The listing builds one solid part. Answer for the finished solid, in the listing's coordinates (mm). A direction names the side the tool comes from. Give positions to 0.01 mm unless a question says otherwise; leave off trailing zeros. Loops run counter-clockwise (first coordinate to the right, second up) from the corner with the lowest first, then second, coordinate; pieces in that order, holes last. Notation, with made-up numbers: M 84,-2 L 110,-2 A19 ccw 110,14 Z; hole C 50,30 d5. An arc over 180 degrees is marked long. Return JSON: item names as keys, results as strings.
from build123d import *

# Parameters (mm, degrees)
SKETCH_2_W      = 230
SKETCH_2_H      = 60
SKETCH_2_R      = 2
EXTRUDE_1_DEPTH = 5


with BuildPart() as part:
    # 草图2 → 凸台-拉伸1 (new body)
    with BuildSketch(Plane.XY):
        Rectangle(SKETCH_2_W, SKETCH_2_H)
        with Locations((-100, 15)):
            Circle(SKETCH_2_R, mode=Mode.SUBTRACT)
        with Locations((100, 15)):
            Circle(SKETCH_2_R, mode=Mode.SUBTRACT)
        with BuildLine():
            Line((-30, 17.5), (30, 17.5))
            ThreePointArc((30, 17.5), (32.5, 15), (30, 12.5))
            Line((30, 12.5), (-30, 12.5))
            ThreePointArc((-30, 12.5), (-32.5, 15), (-30, 17.5))
        make_face(mode=Mode.SUBTRACT)
        with BuildLine():
            Line((40, -23), (100, -23))
            ThreePointArc((100, -23), (102, -25), (100, -27))
            Line((100, -27), (40, -27))
            ThreePointArc((40, -27), (38, -25), (40, -23))
        make_face(mode=Mode.SUBTRACT)
        with BuildLine():
            Line((-100, 10), (-40, 10))
            ThreePointArc((-40, 10), (-38, 8), (-40, 6))
            Line((-40, 6), (-100, 6))
            ThreePointArc((-100, 6), (-102, 8), (-100, 10))
        make_face(mode=Mode.SUBTRACT)
        with BuildLine():
            Line((-100, -10), (-40, -10))
            ThreePointArc((-40, -10), (-38, -8), (-40, -6))
            Line((-40, -6), (-100, -6))
            ThreePointArc((-100, -6), (-102, -8), (-100, -10))
        make_face(mode=Mode.SUBTRACT)
        with BuildLine():
            Line((100, -10), (40, -10))
            ThreePointArc((40, -10), (38, -8), (40, -6))
            Line((40, -6), (100, -6))
            ThreePointArc((100, -6), (102, -8), (100, -10))
        make_face(mode=Mode.SUBTRACT)
        with BuildLine():
            Line((100, 10), (40, 10))
            ThreePointArc((40, 10), (38, 8), (40, 6))
            Line((40, 6), (100, 6))
            ThreePointArc((100, 6), (102, 8), (100, 10))
        make_face(mode=Mode.SUBTRACT)
        with BuildLine():
            Line((-102.1, -17.5), (-102.1, -14.5))
            ThreePointArc((-102.1, -14.5), (-100, -12.4), (-97.9, -14.5))
            Line((-97.9, -14.5), (-97.9, -17.5))
            ThreePointArc((-97.9, -17.5), (-100, -19.6), (-102.1, -17.5))
        make_face(mode=Mode.SUBTRACT)
        with BuildLine():
            Line((102.1, -17.5), (102.1, -14.5))
            ThreePointArc((102.1, -14.5), (100, -12.4), (97.9, -14.5))
            Line((97.9, -14.5), (97.9, -17.5))
            ThreePointArc((97.9, -17.5), (100, -19.6), (102.1, -17.5))
        make_face(mode=Mode.SUBTRACT)
        with BuildLine():
            Line((-30, -17.5), (30, -17.5))
            ThreePointArc((30, -17.5), (32.5, -15), (30, -12.5))
            Line((30, -12.5), (-30, -12.5))
            ThreePointArc((-30, -12.5), (-32.5, -15), (-30, -17.5))
        make_face(mode=Mode.SUBTRACT)
        with BuildLine():
            Line((-40, -23), (-100, -23))
            ThreePointArc((-100, -23), (-102, -25), (-100, -27))
            Line((-100, -27), (-40, -27))
            ThreePointArc((-40, -27), (-38, -25), (-40, -23))
        make_face(mode=Mode.SUBTRACT)
    extrude(amount=EXTRUDE_1_DEPTH)


solid = part.part
(1) A tool of negligible diameter and unlimited length cuts with its end or side. For faces 1 (the cylindrical face through (38, -8, 2)), 2 (the flat face through (-115, 0, 2)), from which of +Z, -Z, +X, -X, +Y, -Y can it reach the whole face along a straight path? Write none if from no direction.
Values follow:
{"face 1": "+Z, -Z", "face 2": "+Z, -Z, -X, +Y, -Y"}
(2) The part is cut by section C-C (z = 3.2). Give the number of separate pieces and of enclosed holes in the cut face, and give its area (3 significant figures).
Values follow:
{"separate pieces": "1", "enclosed holes": "12", "area": "11,600 mm²"}
(3) Straight lines are drawn through the part: line 1 along Y through (x, z) = (-63, 2.95); line 2 along Y through (x, z) = (-100, 1.1); line 3 along X through (y, z) = (-8, 3.2). For each, find the intervals that lie inside material, in ascending order.
Values follow:
{"line 1": "-30 to -27, -23 to -10, -6 to 6, 10 to 30", "line 2": "-30 to -27, -23 to -19.6, -12.4 to -10, -6 to 6, 10 to 13, 17 to 30", "line 3": "-115 to -102, -38 to 38, 102 to 115"}
(4) The part is cut by section A-A (x = 51). Determine the outline of the cut face in (y, z).
Values follow:
{"outline": "M -30,0 L -27,0 L -27,5 L -30,5 Z; M -23,0 L -10,0 L -10,5 L -23,5 Z; M -6,0 L 6,0 L 6,5 L -6,5 Z; M 10,0 L 30,0 L 30,5 L 10,5 Z"}
(5) The part is cut by section B-B (y = -25). Determine the outline of the cut face in (x, z), and give its area (3 significant figures).
Values follow:
{"outline": "M -115,0 L -102,0 L -102,5 L -115,5 Z; M -38,0 L 38,0 L 38,5 L -38,5 Z; M 102,0 L 115,0 L 115,5 L 102,5 Z", "area": "510 mm²"}
(6) Determine the mould class of faces 3 (the flat face through (-70, 10, 2)), 4 (the cylindrical face through (101.908, 15.601, 2.465)), 5 (the flat face through (-2, 30, 2)), 6 (the flat face through (-2, 0, 0)) for opening direction Y: released by +Y, released by -Y, zero draft, split by the parting line, or undercut.
Values follow:
{"face 3": "undercut", "face 4": "undercut", "face 5": "released by +Y", "face 6": "zero draft"}
